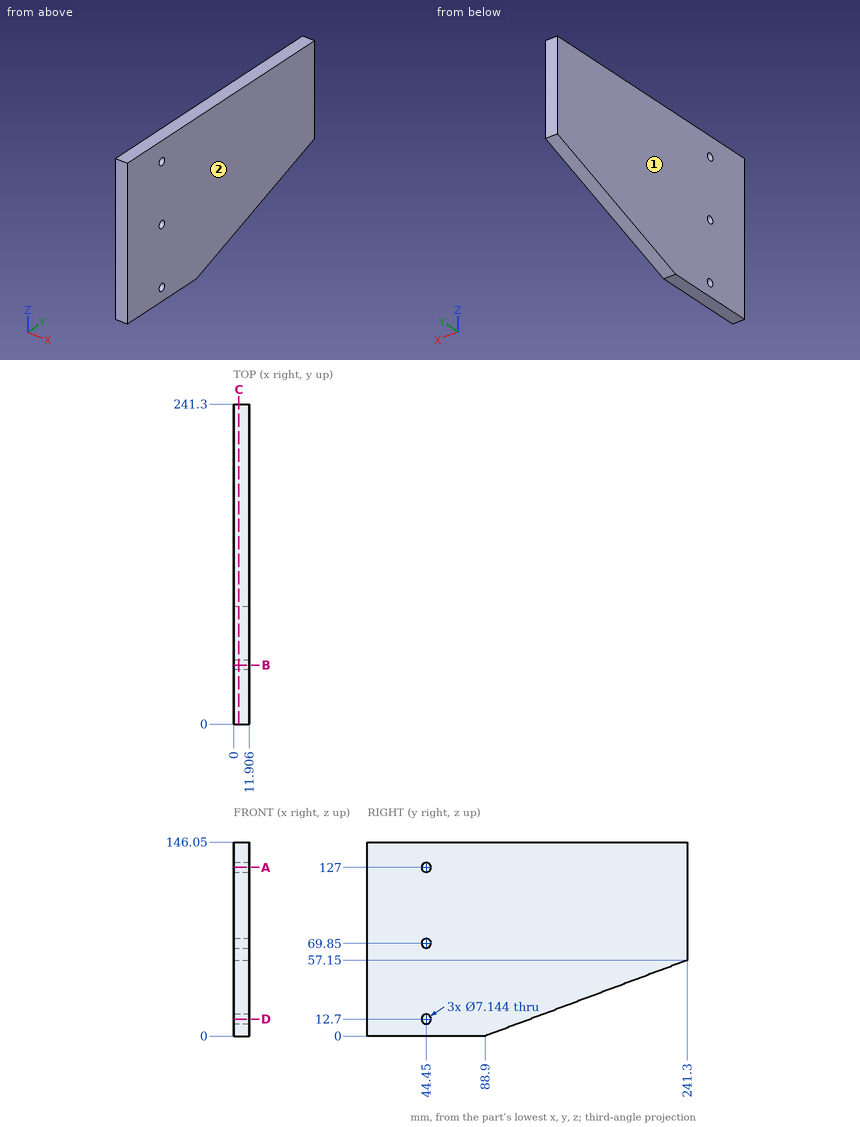
For this review, use the dimensioned drawing (mm, ordinates from the lowest corner) and the shaded views. Round coordinates to 2 decimals unless told otherwise and drop trailing zeros. Loops run counter-clockwise (first coordinate to the right, second up) from the corner with the lowest first, then second, coordinate; pieces in that order, holes last. Notation, with made-up numbers: M 53,67 L 69,67 A17 cw 69,94 Z; hole C 71,85 d9. An arc over 180 degrees is marked long. Answer as a JSON object with one key per item and string values.
(1) Take a section at B-B on y = 44.45. Give the boundary of the cut face in (x, z).
Resolved:
{"outline": "M 0,0 L 11.91,0 L 11.91,9.13 L 0,9.13 Z; M 0,16.27 L 11.91,16.27 L 11.91,66.28 L 0,66.28 Z; M 0,73.42 L 11.91,73.42 L 11.91,123.43 L 0,123.43 Z; M 0,130.57 L 11.91,130.57 L 11.91,146.05 L 0,146.05 Z"}
(2) Clearance check with a flat-ended pin moving along its axis: P1, Ø6, axis at x = 8.5, z = 114.5, coming from the -Y side. State where the tip first meets the part, or that it passes through.
Resolved:
{"P1": "y = 0"}
(3) Take a section at A-A on z = 127. Give the boundary of the cut face in (x, y).
Resolved:
{"outline": "M 0,0 L 11.91,0 L 11.91,40.88 L 0,40.88 Z; M 0,48.02 L 11.91,48.02 L 11.91,241.3 L 0,241.3 Z"}
(4) To check wall thickness, follow line 1 along Y through (x, z) = (5.75, 69.85); line 2 along Z through (x, y) = (6.25, 176); line 3 along Z through (x, y) = (7.5, 116). State the ranges of each line that lie inside material, in increasing order.
Resolved:
{"line 1": "0 to 40.88, 48.02 to 241.3", "line 2": "32.66 to 146.05", "line 3": "10.16 to 146.05"}
(5) Take a section at D-D on z = 12.7. Give the boundary of the cut face in (x, y), and give its area (3 significant figures).
Resolved:
{"outline": "M 0,0 L 11.91,0 L 11.91,40.88 L 0,40.88 Z; M 0,48.02 L 11.91,48.02 L 11.91,122.77 L 0,122.77 Z", "area": "1,380 mm²"}
(6) Draft analysis for pull direction X (two halves, no side actions). For the marked faces 1 and 2, state which applies: released by +X, released by -X, zero draft, split by the parting line, or undercut.
Resolved:
{"face 1": "released by -X", "face 2": "released by +X"}
(7) Take a section at C-C on x = 4. Give the boundary of the cut face in (y, z).
Resolved:
{"outline": "M 0,0 L 88.9,0 L 241.3,57.15 L 241.3,146.05 L 0,146.05 Z; hole C 44.45,12.7 d7.14; hole C 44.45,69.85 d7.14; hole C 44.45,127 d7.14"}
